Read the model definition and answer for the solid it produces. Units are mm, in the model's axes. A direction names the side the tool comes from. Coordinates: 2 decimals unless noted, no trailing zeros. Order: outer loops, then holes, each group sorted by start corner. A loop starts at its lowest first (then second) coordinate and runs counter-clockwise, first axis right, second up. Notation, with made-up numbers: M 38,16.5 L 51,16.5 A26 cw 51,47.5 Z; hole C 51,87 d10. An arc over 180 degrees is marked long. Use a Markdown table: item, result. Add a question column.
1) Find section D-D on y = 181. Write down the section's boundary in (x, z).
2) Find section C-C on x = -52. Write down the section's boundary in (y, z), plus the area to 3 significant figures.
3) Find section B-B on z = 16.5. Write down the section's boundary in (x, y).
4) For faces 1 (the face through (-3.757, 101.14, -100.023)), 2 (the face through (8, 199, -123.52)), 3 (the face through (8, 232, -123.52)), 4 (the face through (8, 216, -174.32)), 5 (the face through (31.671, 215, -99)), determine the directions among +Z, -Z, +X, -X, +Y, -Y from which every point of the face is accessible in a straight line to the end or side of a thin tool.
5) Each of these flat-tipped pins is pushed along its axis until it touches: pin 1 Ø3 at (x, y) = (10, 232) entering from +Z; pin 2 Ø1.9 at (x, y) = (-13.5, 210.5) entering from -Z; pin 3 Ø1.5 at (x, z) = (-56.5, -113) entering from +Y; pin 4 Ø5 at (y, z) = (194, -114.5) entering from -X. Where does it stop, or does it pass through?
6) Find section A-A on z = -82. Write down the section's boundary in (x, y).
7) Find the intervals of material crossed by probe 1 along Y at (x, z) = (31, -106); probe 2 along Y at (x, z) = (-10.5, 15); probe 3 along Y at (x, z) = (5, -168.5), in increasing order. Write a range as [from, to].
8) The mould has two halves that part along Z. Classify faces 6 (the face through (-16.329, 215, -99)), 7 (the face through (7, 215, -75.52)), 8 (the face through (4.92, 1.25, -249.49)), 9 (the face through (2, 202.54, -89)): released by +Z, released by -Z, zero draft, split by the parting line, or undercut.
from build123d import *

# Parameters (mm, degrees)
BOSS_EXTRUDE1_DEPTH = 2.54
SKETCH2_R           = 11.439475367
BOSS_EXTRUDE2_DEPTH = 200
SKETCH3_W           = 48.000000012
SKETCH3_H           = 48.000000012
BOSS_EXTRUDE3_DEPTH = 25.4
SKETCH4_R           = 22.499999958
BOSS_EXTRUDE4_DEPTH = 50.8


with BuildPart() as part:
    # Sketch1 → Boss-Extrude1 (new body)
    with BuildSketch(Plane(origin=(0, 0, 0), x_dir=(1, 0, 0), z_dir=(0, 1, 0))):
        with BuildLine():
            Line((132.671256636, -150.479823869), (-117.328743364, -150.479823869))
            Line((-117.328743364, -150.479823869), (-117.328743364, 124.520176131))
            ThreePointArc((-117.328743364, 124.520176131), (7.671256636, 249.520176131), (132.671256636, 124.520176131))
            Line((132.671256636, 124.520176131), (132.671256636, -150.479823869))
        make_face()
    extrude(amount=BOSS_EXTRUDE1_DEPTH)

    # Sketch2 → Boss-Extrude2 (add)
    with BuildSketch(Plane(origin=(0, 2.54, 0), x_dir=(1, 0, 0), z_dir=(0, 1, 0))):
        with Locations((7.671256636, 99.520176157)):
            Circle(SKETCH2_R)
    extrude(amount=BOSS_EXTRUDE2_DEPTH)

    # Sketch3 → Boss-Extrude3 (add)
    with BuildSketch(Plane(origin=(0, 202.54, 0), x_dir=(1, 0, 0), z_dir=(0, 1, 0))):
        with Locations((7.671256636, 99.520176157)):
            Rectangle(SKETCH3_W, SKETCH3_H)
    extrude(amount=BOSS_EXTRUDE3_DEPTH)

    # Sketch4 → Boss-Extrude4 (add)
    with BuildSketch(Plane(origin=(0, 0, -123.520176163), x_dir=(-1, 0, 0), z_dir=(0, 0, -1))):
        with Locations((-8.000795549, 216.051385612)):
            Circle(SKETCH4_R)
    extrude(amount=BOSS_EXTRUDE4_DEPTH)


solid = part.part
Check result:
| question | item | result |
|---|---|---|
| 1 | outline | C 7.67,-99.52 d22.88 |
| 2 | outline | M 0,-234.36 L 2.54,-234.36 L 2.54,150.48 L 0,150.48 Z |
| 2 | area | 977 mm2 |
| 3 | outline | M -117.33,0 L 132.67,0 L 132.67,2.54 L -117.33,2.54 Z |
| 4 | face 1 | none |
| 4 | face 2 | +X, -X |
| 4 | face 3 | +Z, +X, -X, +Y |
| 4 | face 4 | -Z, +X, -X, +Y |
| 4 | face 5 | +Z, -Z, +X, +Y |
| 5 | pin 1 | stops at z = -123.52 |
| 5 | pin 2 | stops at z = -174.32 |
| 5 | pin 3 | stops at y = 2.54 |
| 5 | pin 4 | passes through |
| 6 | outline | M -117.33,0 L 132.67,0 L 132.67,2.54 L -117.33,2.54 Z; M -16.33,202.54 L 31.67,202.54 L 31.67,227.94 L -16.33,227.94 Z |
| 7 | probe 1 | y = [0, 2.54], [202.54, 227.94] |
| 7 | probe 2 | y = [0, 2.54] |
| 7 | probe 3 | y = [0, 2.54], [193.75, 238.35] |
| 8 | face 6 | zero draft |
| 8 | face 7 | released by +Z |
| 8 | face 8 | released by -Z |
| 8 | face 9 | undercut |
